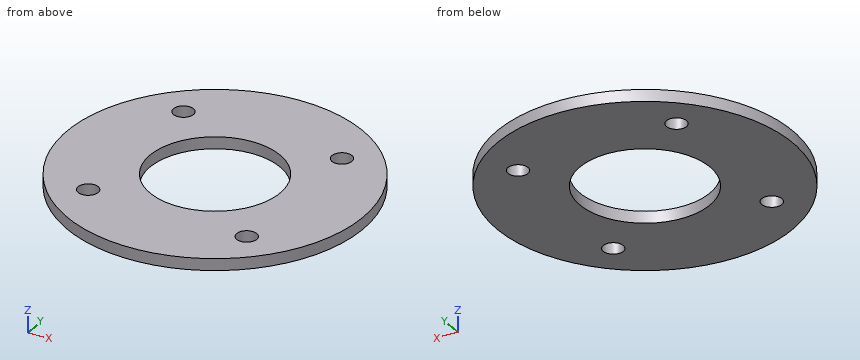
from build123d import *

# Parameters (mm, degrees)
BOSS_EXTRU_1_DEPTH      = 2
BOSS_EXTRU_1_DEPTH_BACK = 0.0001
ESQUISSE1_R             = 25
ESQUISSE1_R_2           = 1.7
ESQUISSE2_R             = 11
ENL_V_MAT_EXTRU_1_DEPTH = 10


with BuildPart() as part:
    # Esquisse1 → Boss.-Extru.1 (new, two sides: drawn at the far end of the back side and taken through both)
    with BuildSketch(Plane.XY.offset(-BOSS_EXTRU_1_DEPTH_BACK)):
        Circle(ESQUISSE1_R)
        with Locations((-13.435028843, 13.435028843)):
            Circle(ESQUISSE1_R_2, mode=Mode.SUBTRACT)
        with Locations((13.435028843, 13.435028843)):
            Circle(ESQUISSE1_R_2, mode=Mode.SUBTRACT)
        with Locations((13.435028843, -13.435028843)):
            Circle(ESQUISSE1_R_2, mode=Mode.SUBTRACT)
        with Locations((-13.435028843, -13.435028843)):
            Circle(ESQUISSE1_R_2, mode=Mode.SUBTRACT)
    extrude(amount=BOSS_EXTRU_1_DEPTH + BOSS_EXTRU_1_DEPTH_BACK)

    # Esquisse2 → Enlèv. mat.-Extru.1 (cut)
    with BuildSketch(Plane(origin=(0, 0, -0.0001), x_dir=(-1, 0, 0), z_dir=(0, 0, -1))):
        Circle(ESQUISSE2_R)
    extrude(amount=-ENL_V_MAT_EXTRU_1_DEPTH, mode=Mode.SUBTRACT)


solid = part.part
Read the model definition and answer for the solid it produces. Units are mm, in the model's axes. Coordinates: 2 decimals unless noted, no trailing zeros. Loops run counter-clockwise (first coordinate to the right, second up) from the corner with the lowest first, then second, coordinate; pieces in that order, holes last.
Q1. Each of these flat-tipped pins is pushed along its axis until it touches: pin 1 Ø3 at (x, y) = (-13.44, -13.44) entering from -Z; pin 2 Ø4.5 at (x, y) = (13.44, 13.44) entering from -Z. Where does it stop, or does it pass through?
Q2. The part is cut by section D-D on z = 1.55. Write down the section's boundary in (x, y), and give its area (3 significant figures).
Q3. The part is cut by section A-A on x = 0. Write down the section's boundary in (y, z), and give its area (3 significant figures).
Q4. The part is cut by section C-C on x = 14. Write down the section's boundary in (y, z).
Q5. Consider probe 1 along X at (y, z) = (-13, 1.6); probe 2 along Y at (x, z) = (-14, 1.8). Determine where each line is inside the solid, lowest interval first.
Results below:
1. pin 1: passes through
1. pin 2: stops at z = 0
2. outline: circle Ø50 at (0, 0); hole circle Ø3.4 at (-13.44, -13.44); hole circle Ø3.4 at (-13.44, 13.44); hole circle Ø22 at (0, 0); hole circle Ø3.4 at (13.44, -13.44); hole circle Ø3.4 at (13.44, 13.44)
2. area: 1,550 mm2
3. outline: (-25, 0) - (-11, 0) - (-11, 2) - (-25, 2) - close; (11, 0) - (25, 0) - (25, 2) - (11, 2) - close
3. area: 56.0 mm2
4. outline: (-20.71, 0) - (-15.04, 0) - (-15.04, 2) - (-20.71, 2) - close; (-11.83, 0) - (11.83, 0) - (11.83, 2) - (-11.83, 2) - close; (15.04, 0) - (20.71, 0) - (20.71, 2) - (15.04, 2) - close
5. probe 1: x = -21.35 to -15.08, -11.79 to 11.79, 15.08 to 21.35
5. probe 2: y = -20.71 to -15.04, -11.83 to 11.83, 15.04 to 20.71
